Work out the finished part from the listing and answer in its coordinate system (mm). Round coordinates to 2 decimals unless told otherwise and drop trailing zeros. Write each loop counter-clockwise with the first axis right and the second up, starting at its lowest first coordinate (ties: lowest second). Pieces come first, ordered by that corner, then holes.
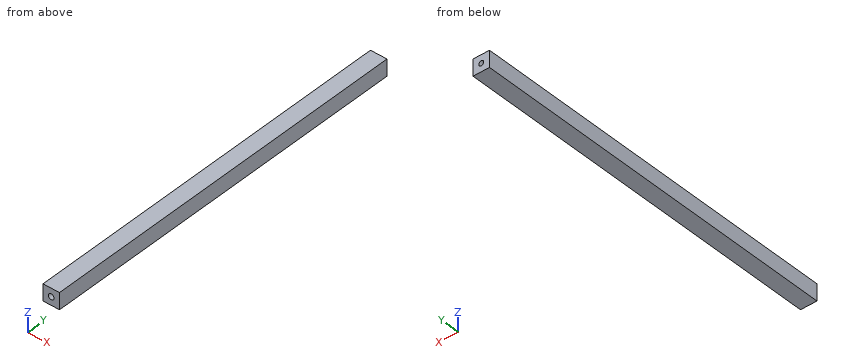
from build123d import *

# Parameters (mm, degrees)
SKETCH_1_W             = 20
SKETCH_1_H             = 460
EXTRUDE_1_DEPTH        = 20
CUT_EXTRUDE_1_DEPTH    = 400
HOLE_WIZARD_M8_1_D     = 6.8
HOLE_WIZARD_M8_1_DEPTH = 19.75
HOLE_WIZARD_M8_1_TIP   = 2.042926105


with BuildPart() as part:
    # 草图1 → 凸台-拉伸1 (new body)
    with BuildSketch(Plane.XY):
        with Locations((10, 230)):
            Rectangle(SKETCH_1_W, SKETCH_1_H)
    extrude(amount=EXTRUDE_1_DEPTH)

    # 草图2 → 切除-拉伸1 (cut)
    with BuildSketch(Plane(origin=(0, 460, 0), x_dir=(1, 0, 0), z_dir=(0, 1, 0))):
        with BuildLine():
            ThreePointArc((13, -10), (10, -7), (7, -10))
            Line((7, -10), (13, -10))
        make_face()
        with BuildLine():
            Line((13, -10), (7, -10))
            ThreePointArc((7, -10), (10, -13), (13, -10))
        make_face()
    extrude(amount=-CUT_EXTRUDE_1_DEPTH, mode=Mode.SUBTRACT)

    # M8 螺纹孔1
    with Locations(Plane(origin=(0, 0, 0), x_dir=(-1, 0, 0), z_dir=(0, -1, 0))):
        with Locations((-10, -10)):
            Hole(HOLE_WIZARD_M8_1_D / 2, depth=HOLE_WIZARD_M8_1_DEPTH)
            with Locations((0, 0, -(HOLE_WIZARD_M8_1_DEPTH + HOLE_WIZARD_M8_1_TIP / 2))):  # 118° drill point
                Cone(0, HOLE_WIZARD_M8_1_D / 2, HOLE_WIZARD_M8_1_TIP, mode=Mode.SUBTRACT)


solid = part.part
Q1. Find section A-A (y = 189). Determine the outline of the cut face in (x, z), plus the area to 3 significant figures.
Q2. Find the intervals of material crossed by L1, parallel to Z at x = 10, y = 278.5; L2, parallel to Z at x = 10, y = 6, in increasing order.
Q3. Given pin 1 (2 mm diameter, centred on y = 146.5, z = 6.5, fed in from -X); pin 2 (5.5 mm diameter, centred on x = 10, z = 10, fed in from +Y), each flat-ended and moving along its own axis, determine where each tip first touches the part or whether it passes through.
Report:
1. outline: (0, 0) - (20, 0) - (20, 20) - (0, 20) - close; hole circle Ø6 at (10, 10)
1. area: 372 mm2
2. L1: z = 0 to 7, 13 to 20
2. L2: z = 0 to 6.6, 13.4 to 20
3. pin 1: stops at x = 0
3. pin 2: stops at y = 60
